Read the model definition and answer for the solid it produces. Units are mm, in the model's axes. A direction names the side the tool comes from. Coordinates: 2 decimals unless noted, no trailing zeros. Write each loop counter-clockwise with the first axis right and the second up, starting at its lowest first coordinate (ties: lowest second). Pieces come first, ordered by that corner, then holes.
Item 1: A tool of negligible diameter and unlimited length cuts with its end or side. For faces 1 (the face through (-13, -6, 0)), 2 (the face through (-29.31, 5.96, 1.23)), 3 (the face through (35, 5, -1)), 4 (the face through (29.19, 6.04, 1.23)), from which of +Z, -Z, +X, -X, +Y, -Y can it reach the whole face along a straight path? Write none if from no direction.
Item 2: Section D-D (y = -1) is taken. Give the vertices of the cut face in (x, z), then the cut area to 3 significant figures.
Item 3: Section A-A (z = 0.7) is taken. Give the vertices of the cut face in (x, y).
Item 4: Each of these flat-tipped pins is pushed along its axis until it touches: P1, Ø1.2, axis at y = 0.5, z = 1.5, coming from the -X side; P2, Ø2, axis at x = -3, z = 1.5, coming from the -Y side. Where does it stop, or does it pass through?
Item 5: Straight lines are drawn through the part: probe 1 along X at (y, z) = (0, -1.15); probe 2 along X at (y, z) = (0, 1.55); probe 3 along Y at (x, z) = (25, -0.5). For each, find the intervals that lie inside material, in ascending order.
Item 6: Section B-B (x = -21.5) is taken. Give the vertices of the cut face in (y, z), then the cut area to 3 significant figures.
Item 7: Section C-C (y = 15.3) is taken. Give the vertices of the cut face in (x, z), then the cut area to 3 significant figures.
Item 8: Determine the mould class of faces 5 (the face through (31.99, 17.15, -1.27)), 6 (the face through (-33.5, 0, 1)), 7 (the face through (23.4, 14.1, -1.2)), 8 (the face through (7.5, 0.1, 0)) for opening direction X: released by +X, released by -X, zero draft, split by the parting line, or undercut.
from build123d import *

# Parameters (mm, degrees)
BOSS_EXTRUDE1_DEPTH     = 2.5
SKETCH2_W               = 70
SKETCH2_H               = 30
BOSS_EXTRUDE2_DEPTH     = 2.5
SKETCH3_R               = 2
CUT_EXTRUDE1_DEPTH      = 2.5
FILLET1_R               = 10
SKETCH4_R               = 2.5
SKETCH4_W               = 20
SKETCH4_H               = 12
CUT_EXTRUDE2_DEPTH      = 3.5
CUT_EXTRUDE2_DEPTH_BACK = 3.5


with BuildPart() as part:
    # Sketch1 → Boss-Extrude1 (new body)
    with BuildSketch(Plane.XY):
        Polygon((-33.5, 3), (-25, 9), (25, 9), (33.5, 3), (33.5, -3), (25, -9), (-25, -9), (-33.5, -3), align=None)
    extrude(amount=BOSS_EXTRUDE1_DEPTH)

    # Sketch2 → Boss-Extrude2 (add)
    with BuildSketch(Plane.XY):
        with Locations((0, 5)):
            Rectangle(SKETCH2_W, SKETCH2_H)
    extrude(amount=-BOSS_EXTRUDE2_DEPTH)

    # Sketch3 → Cut-Extrude1 (cut)
    with BuildSketch(Plane.XY):
        with Locations((25, 15.3)):
            Circle(SKETCH3_R)
    extrude(amount=-CUT_EXTRUDE1_DEPTH, mode=Mode.SUBTRACT)

    # Fillet1
    fillet1_edges = [part.edges().sort_by_distance(p)[0] for p in [
        (35, 20, -1.25),
        (35, -10, -1.25),
        (-35, -10, -1.25),
        (-35, 20, -1.25),
    ]]
    fillet(fillet1_edges, radius=FILLET1_R)

    # Sketch4 → Cut-Extrude2 (cut, two sides)
    with BuildSketch(Plane.XY) as cut_extrude2_sk:
        with Locations((10, 0)):
            Circle(SKETCH4_R)
        with Locations((20, 0)):
            Circle(SKETCH4_R)
        with Locations((-12.5, 0)):
            Rectangle(SKETCH4_W, SKETCH4_H)
    extrude(amount=CUT_EXTRUDE2_DEPTH, mode=Mode.SUBTRACT)
    extrude(cut_extrude2_sk.sketch, amount=-CUT_EXTRUDE2_DEPTH_BACK, mode=Mode.SUBTRACT)


solid = part.part
Established:
1. face 1: +Z, -Z
1. face 2: +Z, -X, +Y
1. face 3: +Z, -Z, +X, +Y, -Y
1. face 4: +Z, +X, +Y
2. outline: (-34.95, -2.5) - (-22.5, -2.5) - (-22.5, 2.5) - (-33.5, 2.5) - (-33.5, 0) - (-34.95, 0) - close; (-2.5, -2.5) - (7.71, -2.5) - (7.71, 2.5) - (-2.5, 2.5) - close; (12.29, -2.5) - (17.71, -2.5) - (17.71, 2.5) - (12.29, 2.5) - close; (22.29, -2.5) - (34.95, -2.5) - (34.95, 0) - (33.5, 0) - (33.5, 2.5) - (22.29, 2.5) - close
2. area: 196 mm2
3. outline: (-33.5, -3) - (-25, -9) - (25, -9) - (33.5, -3) - (33.5, 3) - (25, 9) - (-25, 9) - (-33.5, 3) - close; hole (-22.5, -6) - (-2.5, -6) - (-2.5, 6) - (-22.5, 6) - close; hole circle Ø5 at (10, 0); hole circle Ø5 at (20, 0)
4. P1: stops at x = -33.5
4. P2: stops at y = -9
5. probe 1: x = -35 to -22.5, -2.5 to 7.5, 12.5 to 17.5, 22.5 to 35
5. probe 2: x = -33.5 to -22.5, -2.5 to 7.5, 12.5 to 17.5, 22.5 to 33.5
5. probe 3: y = -10 to 13.3, 17.3 to 20
6. outline: (-10, -2.5) - (-6, -2.5) - (-6, 2.5) - (-9, 2.5) - (-9, 0) - (-10, 0) - close; (6, -2.5) - (20, -2.5) - (20, 0) - (9, 0) - (9, 2.5) - (6, 2.5) - close
6. area: 60.0 mm2
7. outline: (-33.48, -2.5) - (23, -2.5) - (23, 0) - (-33.48, 0) - close; (27, -2.5) - (33.48, -2.5) - (33.48, 0) - (27, 0) - close
7. area: 157 mm2
8. face 5: released by +X
8. face 6: released by -X
8. face 7: undercut
8. face 8: undercut
